Autodesk Inventor part; units mm, degrees
ref_plane "YZ Plane" through (0, 0, 0) normal (1, 0, 0) x (0, 1, 0)
ref_plane "XZ Plane" through (0, 0, 0) normal (0, 1, 0) x (-1, 0, 0)
ref_plane "XY Plane" through (0, 0, 0) normal (0, 0, 1) x (1, 0, 0)
sketch "Sketch1" plane through (0, 0, 0) normal (1, 0, 0) x (0, 1, 0)
  line L0 (0, 0) -> (25.4, 0)
  line L1 (25.4, 0) -> (25.4, 25.4)
  line L2 (25.4, 25.4) -> (0, 25.4)
  line L3 (0, 25.4) -> (0, 0)
  line L4 (22.86, 22.86) -> (22.86, 2.54)
  line L5 (22.86, 2.54) -> (2.54, 2.54)
  line L6 (2.54, 2.54) -> (2.54, 22.86)
  line L7 (2.54, 22.86) -> (22.86, 22.86)
  dimension "d0" = 2.54
  dimension "d1" = 25.4
  dimension "d2" = 25.4
extrude "Extrusion1" add sketch "Sketch1" along normal blind 457.2
sketch "Sketch2" plane through (0, 0, 25.4) normal (0, 0, 1) x (1, 0, 0)
  line L0 (15.875, 15.875) -> (441.325, 15.875)
  line L1 (444.5, 12.7) -> (444.5, 12.7)
  line L2 (441.325, 9.525) -> (15.875, 9.525)
  line L3 (12.7, 12.7) -> (12.7, 12.7)
  line L4 (457.2, 25.4) -> (457.2, 0)
  line L5 (0, 25.4) -> (0, 0)
  line L6 (0, 25.4) -> (457.2, 25.4)
  arc A0 (15.875, 15.875) -> (12.7, 12.7) centre (15.875, 12.7) ccw
  arc A1 (12.7, 12.7) -> (15.875, 9.525) centre (15.875, 12.7) ccw
  arc A2 (444.5, 12.7) -> (441.325, 15.875) centre (441.325, 12.7) ccw
  arc A3 (441.325, 9.525) -> (444.5, 12.7) centre (441.325, 12.7) ccw
  point P0 (12.7, 15.875)
  point P1 (12.7, 9.525)
  dimension "d5" = 6.35
  dimension "d6" = 12.7
  dimension "d7" = 12.7
  dimension "d8" = 9.525
  dimension "d9" = 3.175
extrude "Extrusion2" cut sketch "Sketch2" against normal blind 457.2
properties part number "Rail"
The model under review builds one solid part; all positions refer to its coordinate system, in mm. A direction names the side the tool comes from. Round coordinates to 2 decimals unless told otherwise and drop trailing zeros. Loops run counter-clockwise (first coordinate to the right, second up) from the corner with the lowest first, then second, coordinate; pieces in that order, holes last.
1) The part is to be moulded in two halves that separate along Z. For faces 3 (the face through (225, 8, 2.54)), 4 (the face through (225, 8, 22.86)), 5 (the face through (225, 7, 25.4)), 6 (the face through (225, 18, 0)), say which applies: pulls with the +Z half, pulls with the -Z half, needs draft (parallel to the pull), parting line crosses it, or undercut.
Values follow:
face 3: undercut
face 4: undercut
face 5: pulls with the +Z half
face 6: pulls with the -Z half
2) Tool access review of faces 1 (the face through (225, 22.86, 13)), 2 (the face through (457.2, 24, 13)): name each direction out of +Z, -Z, +X, -X, +Y, -Y from which nothing blocks a thin tool from reaching the whole face with its end or side.
Values follow:
face 1: +X, -X
face 2: +Z, -Z, +X, +Y, -Y
3) Consider section A-A on z = 11.75. State the section outline as (x, y) points, then the cut area to 3 significant figures.
Values follow:
outline: (0, 0) - (457.2, 0) - (457.2, 2.54) - (0, 2.54) - close; (0, 22.86) - (457.2, 22.86) - (457.2, 25.4) - (0, 25.4) - close
area: 2,320 mm2
4) Consider section B-B on x = 171. State the section outline as (y, z) points (3 decimals), then the cut area to 3 significant figures.
Values follow:
outline: (0, 0) - (9.525, 0) - (9.525, 2.54) - (2.54, 2.54) - (2.54, 22.86) - (9.525, 22.86) - (9.525, 25.4) - (0, 25.4) - close; (15.875, 0) - (25.4, 0) - (25.4, 25.4) - (15.875, 25.4) - (15.875, 22.86) - (22.86, 22.86) - (22.86, 2.54) - (15.875, 2.54) - close
area: 200 mm2
5) Wall thickness on line 1 along Y through (x, z) = (271, 16.75); line 2 along Y through (x, z) = (64, 1.75) (3 decimals): over which ranges is each line inside the solid? List them lowest first.
Values follow:
line 1: y = 0 to 2.54, 22.86 to 25.4
line 2: y = 0 to 9.525, 15.875 to 25.4
